The listing builds one solid part. Answer for the finished solid, in the listing's coordinates (mm). A direction names the side the tool comes from. Round coordinates to 2 decimals unless told otherwise and drop trailing zeros. Order: outer loops, then holes, each group sorted by start corner. A loop starts at its lowest first (then second) coordinate and runs counter-clockwise, first axis right, second up. Notation, with made-up numbers: (-19, 24.5) - (-12, 24.5) arc R33 ccw to (-12, 61.5) - close; hole circle Ø8 at (24.5, 49.5). An arc over 180 degrees is marked (long way). Use CSV: the item, a comma, the result in double quotes. Start each with the question number.
Item 1: Straight lines are drawn through the part: line 1 along Y through (x, z) = (-38.1, 0.6); line 2 along Y through (x, z) = (-321, 0.25); line 3 along X through (y, z) = (14, 0.9). For each, find the intervals that lie inside material, in ascending order. Write a range as [from, to].
Item 2: For faces 3 (the cylindrical face through (-42.628, 45.846, 1.565)), 4 (the flat face through (-206, 39, 0)), determine the directions among +Z, -Z, +X, -X, +Y, -Y from which every point of the face is accessible in a straight line to the end or side of a thin tool.
Item 3: Find section C-C, the plane z = 0.95. Count the separate pieces of the cut face and the enclosed holes in it, plus the area to 3 significant figures.
Item 4: A flat-ended cylindrical pin translates along its axis: P1, Ø1.5, axis at x = -213.5, y = 62, coming from the -Z side. Find the tip coordinate at first contact, or state that the pin passes through.
Item 5: Find section B-B, the plane x = -240. Give the vertices of the cut face in (y, z) (3 decimals).
Item 6: Find section A-A, the plane x = -38.1. Give the vertices of the cut face in (y, z) (3 decimals).
Item 7: Determine the mould class of faces 1 (the flat face through (-148.63, 23.5, 1.57)), 2 (the flat face through (-206, 39, 3.175)) for opening direction X: +X half, -X half, draft (parallel to the pull), parting line (faces both ways), or undercut.
Autodesk Inventor part; units mm, degrees
ref_plane "YZ Plane" through (0, 0, 0) normal (1, 0, 0) x (0, 1, 0)
ref_plane "XZ Plane" through (0, 0, 0) normal (0, 1, 0) x (-1, 0, 0)
ref_plane "XY Plane" through (0, 0, 0) normal (0, 0, 1) x (1, 0, 0)
sketch "Sketch1" plane through (0, 0, 0) normal (0, 0, 1) x (1, 0, 0)
  line L0 (-125.1151, 28.732) -> (-166.2826, 33.9736)
  arc A0 (-123.528, 23.1069) -> (-125.1151, 28.732) centre (-125.5161, 25.5824) ccw
  arc A1 (-123.528, 23.1069) -> (-126.0625, 20.4145) centre (-115.1699, 12.7) ccw
  arc A2 (-129.3518, 19.1523) -> (-126.0625, 20.4145) centre (-128.6535, 22.2495) ccw
  line L1 (-167.3819, 27.7268) -> (-129.3518, 19.1523)
  arc A3 (-166.2826, 33.9736) -> (-167.3819, 27.7268) centre (-166.6836, 30.824) ccw
  line L2 (-321.3346, 53.089) -> (-381.486, 59.0906)
  arc A4 (-320.2929, 47.0593) -> (-321.3346, 53.089) centre (-321.6498, 49.9297) ccw
  line L3 (-348.7058, 33.6279) -> (-320.2929, 47.0593)
  arc A5 (-352.4725, 34.4311) -> (-348.7058, 33.6279) centre (-350.0627, 36.4983) ccw
  arc A6 (-352.4725, 34.4311) -> (-373.8567, 40.9528) centre (-368.3, 20.8534) ccw
  arc A7 (-377.4306, 42.3884) -> (-373.8567, 40.9528) centre (-374.7028, 44.013) ccw
  line L4 (-384.529, 54.3066) -> (-377.4306, 42.3884)
  arc A8 (-381.486, 59.0906) -> (-384.529, 54.3066) centre (-381.8012, 55.9313) ccw
  arc A9 (-390.525, 12.7) -> (-388.6543, 16.3183) centre (-391.7533, 15.6278) ccw
  arc A10 (-393.7, 15.875) -> (-390.525, 12.7) centre (-390.525, 15.875) ccw
  line L5 (-393.7, 45.7598) -> (-393.7, 15.875)
  arc A11 (-387.7972, 47.3844) -> (-393.7, 45.7598) centre (-390.525, 45.7598) ccw
  line L6 (-382.8862, 39.139) -> (-387.7972, 47.3844)
  arc A12 (-383.3263, 35.3128) -> (-382.8862, 39.139) centre (-385.6141, 37.5143) ccw
  arc A13 (-383.3263, 35.3128) -> (-388.6543, 16.3183) centre (-368.3, 20.8534) ccw
  line L7 (-12.7, 38.8139) -> (-12.7, 60.325)
  arc A14 (-18.3444, 36.8183) -> (-12.7, 38.8139) centre (-15.875, 38.8139) ccw
  arc A15 (-18.3444, 36.8183) -> (-61.9536, 29.5806) centre (-38.1, 20.8534) ccw
  arc A16 (-65.3364, 27.5219) -> (-61.9536, 29.5806) centre (-64.9353, 30.6715) ccw
  line L8 (-282.7016, 55.1979) -> (-65.3364, 27.5219)
  arc A17 (-285.3624, 57.5073) -> (-282.7016, 55.1979) centre (-282.3006, 58.3475) ccw
  arc A18 (-285.3624, 57.5073) -> (-285.9117, 59.1048) centre (-298.2343, 53.975) ccw
  arc A19 (-282.9805, 63.5) -> (-285.9117, 59.1048) centre (-282.9805, 60.325) ccw
  line L9 (-15.875, 63.5) -> (-282.9805, 63.5)
  arc A20 (-12.7, 60.325) -> (-15.875, 63.5) centre (-15.875, 60.325) ccw
  arc A21 (-343.1641, 29.2238) -> (-341.9094, 23.18) centre (-341.8072, 26.3534) ccw
  line L10 (-310.6679, 44.5855) -> (-343.1641, 29.2238)
  arc A22 (-307.1824, 44.0709) -> (-310.6679, 44.5855) centre (-309.3109, 41.715) ccw
  arc A23 (-307.1824, 44.0709) -> (-287.3417, 46.2605) centre (-298.2343, 53.975) ccw
  arc A24 (-284.0524, 47.5227) -> (-287.3417, 46.2605) centre (-284.7507, 44.4255) ccw
  line L11 (-181.0291, 24.2944) -> (-284.0524, 47.5227)
  arc A25 (-181.8296, 18.0238) -> (-181.0291, 24.2944) centre (-181.7274, 21.1971) ccw
  line L12 (-341.9094, 23.18) -> (-181.8296, 18.0238)
  arc A26 (-103.4554, 19.0977) -> (-104.4707, 20.6804) centre (-115.1699, 12.7) ccw
  arc A27 (-101.5246, 25.7283) -> (-104.4707, 20.6804) centre (-101.9257, 22.5787) ccw
  line L13 (-92.5499, 24.5856) -> (-101.5246, 25.7283)
  arc A28 (-92.6169, 18.2787) -> (-92.5499, 24.5856) centre (-92.9509, 21.436) ccw
  line L14 (-100.3348, 17.4622) -> (-92.6169, 18.2787)
  arc A29 (-103.4554, 19.0977) -> (-100.3348, 17.4622) centre (-100.6689, 20.6195) ccw
  circle A30 centre (-298.2343, 53.975) radius 6.9977
  circle A31 centre (-115.1699, 12.7) radius 6.9977
  circle A32 centre (-38.1, 20.8534) radius 14.5034
  circle A33 centre (-368.3, 20.8534) radius 14.5034
  line L15 (0, 76.2) -> (0, 0)
  line L16 (0, 76.2) -> (-406.4, 76.2)
  line L17 (-406.4, 76.2) -> (-406.4, 0)
  line L18 (0, 0) -> (-406.4, 0)
  point P0 (0, 30.4367)
extrude "Extrusion1" add sketch "Sketch1" along normal blind 3.175
properties part number "Left left side"
Worked out:
1,line 1,"y = [0, 6.35], [35.36, 46.25], [63.5, 76.2]"
1,line 2,"y = [0, 22.51], [39.7, 46.73], [53.04, 76.2]"
1,line 3,"x = [-406.4, -393.09], [-389.03, -381.08], [-355.52, -122.05], [-108.29, -50.88], [-25.32, 0]"
2,face 3,"+Z, -Z"
2,face 4,"-Z, +X, -X, +Y, -Y"
3,separate pieces,"1"
3,enclosed holes,"10"
3,area,"18,900 mm²"
4,P1,"passes through"
5,outline,"(0, 0) - (19.897, 0) - (19.897, 3.175) - (0, 3.175) - close; (37.59, 0) - (49.761, 0) - (49.761, 3.175) - (37.59, 3.175) - close; (63.5, 0) - (76.2, 0) - (76.2, 3.175) - (63.5, 3.175) - close"
6,outline,"(0, 0) - (6.35, 0) - (6.35, 3.175) - (0, 3.175) - close; (35.357, 0) - (46.253, 0) - (46.253, 3.175) - (35.357, 3.175) - close; (63.5, 0) - (76.2, 0) - (76.2, 3.175) - (63.5, 3.175) - close"
7,face 1,"undercut"
7,face 2,"draft"
